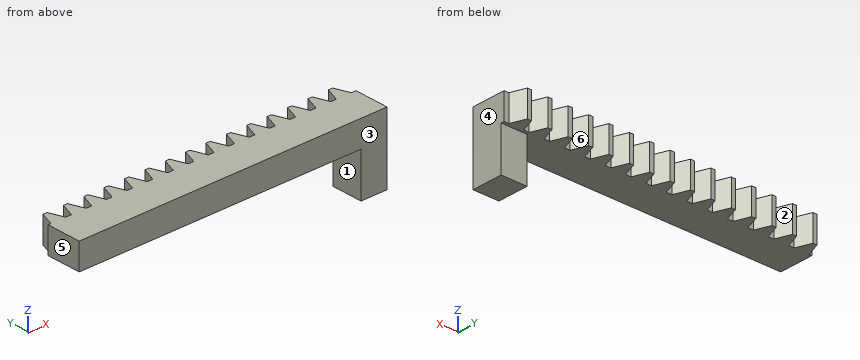
```python
from build123d import *

# Parameters (mm, degrees)
BLANKSKE_W          = 120
BLANKSKE_H          = 16
BLANK_DEPTH         = 8
TOOTHCUTSIM_DEPTH   = 122.326007105
TEETHCUTS_COUNT     = 20
TEETHCUTS_PITCH     = 6.2831853
SKETCH1_W           = 8
SKETCH1_H           = 1
CUT_EXTRUDE1_DEPTH  = 122.326007105
SKETCH2_W           = 13.5
SKETCH2_H           = 9.5
BOSS_EXTRUDE2_DEPTH = 8
CUT_EXTRUDE2_DEPTH  = 123.956293048


with BuildPart() as part:
    # BlankSke → Blank (new body)
    with BuildSketch(Plane.XY):
        with Locations((60, 8)):
            Rectangle(BLANKSKE_W, BLANKSKE_H)
    extrude(amount=-BLANK_DEPTH)

    # TooCutSkeSim → ToothCutSim (cut, through all)
    with BuildSketch(Plane.XY):
        Polygon((0.861870739, 11.5), (-0.861870739, 11.5), (-2.508981637, 16.0254), (2.508981637, 16.0254), align=None)
    toothcutsim = extrude(amount=-TOOTHCUTSIM_DEPTH, mode=Mode.SUBTRACT)

    # TeethCuts: ToothCutSim ×20
    with Locations(*[(i * TEETHCUTS_PITCH, 0, 0) for i in range(1, TEETHCUTS_COUNT)]):
        add(toothcutsim, mode=Mode.SUBTRACT)

    # Sketch1 → Cut-Extrude1 (cut, through all)
    with BuildSketch(Plane(origin=(120, 0, 0), x_dir=(0, 0, -1), z_dir=(1, 0, 0))):
        with Locations((4, 0.5)):
            Rectangle(SKETCH1_W, SKETCH1_H)
    extrude(amount=-CUT_EXTRUDE1_DEPTH, mode=Mode.SUBTRACT)

    # Sketch2 → Boss-Extrude2 (add)
    with BuildSketch(Plane(origin=(120, 0, 0), x_dir=(0, 0, -1), z_dir=(1, 0, 0))):
        with Locations((14.75, 5.75)):
            Rectangle(SKETCH2_W, SKETCH2_H)
    extrude(amount=-BOSS_EXTRUDE2_DEPTH)

    # Sketch3 → Cut-Extrude2 (cut, through all)
    with BuildSketch(Plane.XY):
        with BuildLine():
            Line((0, 1), (0, 11.5))
            ThreePointArc((0, 11.5), (0.43093537, 11.93093537), (0.861870739, 11.5))
            Line((0.861870739, 11.5), (2.499736794, 16))
            Line((2.499736794, 16), (3.783448506, 16))
            Line((3.783448506, 16), (5.421314561, 11.5))
            Line((5.421314561, 11.5), (7.145056039, 11.5))
            Line((7.145056039, 11.5), (8.782922094, 16))
            Line((8.782922094, 16), (10.066633806, 16))
            Line((10.066633806, 16), (11.704499861, 11.5))
            Line((11.704499861, 11.5), (13.428241339, 11.5))
            Line((13.428241339, 11.5), (15.066107394, 16))
            Line((15.066107394, 16), (15.70796325, 16))
            Line((15.70796325, 16), (16.349819106, 16))
            Line((16.349819106, 16), (17.987685161, 11.5))
            Line((17.987685161, 11.5), (19.711426639, 11.5))
            Line((19.711426639, 11.5), (21.349292694, 16))
            Line((21.349292694, 16), (22.633004406, 16))
            Line((22.633004406, 16), (24.270870461, 11.5))
            Line((24.270870461, 11.5), (25.1327412, 11.5))
            Line((25.1327412, 11.5), (25.1327412, 1))
            Line((25.1327412, 1), (17.987685161, 1))
            Line((17.987685161, 1), (15.70796325, 1))
            Line((15.70796325, 1), (6.161314561, 1))
            Line((6.161314561, 1), (0, 1))
        make_face()
    extrude(amount=-CUT_EXTRUDE2_DEPTH, mode=Mode.SUBTRACT)


solid = part.part
```
The listing builds one solid part. Answer for the finished solid, in the listing's coordinates (mm). Face numbers are marked on the shaded views. A direction names the side the tool comes from. Give positions to 0.01 mm unless a question says otherwise; leave off trailing zeros. Order: outer loops, then holes, each group sorted by start corner. A loop starts at its lowest first (then second) coordinate and runs counter-clockwise, first axis right, second up. Notation, with made-up numbers: (15, -6.5) -> (74, -6.5) arc R33 ccw to (74, 24.5) -> close; hole circle Ø8 at (70.25, 8.5). An arc over 180 degrees is marked (long way). Write each question's results on one line, items separated by ' | '.
Q1. The part is cut by section B-B, the plane y = 2.5. Give the vertices of the cut face in (x, z), and give its area (3 significant figures).
Checked values:
outline: (25.13, -8) -> (112, -8) -> (112, -21.5) -> (120, -21.5) -> (120, 0) -> (25.13, 0) -> close | area: 867 mm^2
Q2. Which of the six approach directions +Z, -Z, +X, -X, +Y, -Y give full straight-line access (tool end or side, diameter ignored) to the marked faces 5 and 6?
Checked values:
face 5: +Z, -Z, -X, +Y, -Y | face 6: +Z, -Z, +Y
Q3. Each of these flat-tipped pins is pushed along its axis until it touches: P1, Ø10, axis at x = 35.5, z = -8, coming from the +Y side; P2, Ø4.5, axis at x = 61, y = 8, coming from the -Z side; P3, Ø0.9, axis at x = 113, z = -4.5, coming from the +Y side; P4, Ø2.5, axis at x = 117, z = -14, coming from the +Y side. Where does it stop, or does it pass through?
Checked values:
P1: stops at y = 16 | P2: stops at z = -8 | P3: stops at y = 11.5 | P4: stops at y = 10.5
Q4. The part is cut by section A-A, the plane z = -11. Give the vertices of the cut face in (x, y).
Checked values:
outline: (112, 1) -> (120, 1) -> (120, 10.5) -> (112, 10.5) -> close
Q5. Determine the mould class of the marked faces 1, 2, 3 and 4 for opening direction X: pulls with the +X half, pulls with the -X half, needs draft (parallel to the pull), parting line crosses it, or undercut.
Checked values:
face 1: pulls with the -X half | face 2: undercut | face 3: needs draft | face 4: pulls with the +X half
Q6. Straight lines are drawn through the part: probe 1 along Y at (x, z) = (75, -1); probe 2 along Z at (x, y) = (67, 3.5); probe 3 along X at (y, z) = (6.25, -15.75). For each, find the intervals that lie inside material, in ascending order. Write a range as from..to.
Checked values:
probe 1: y = 1..11.5 | probe 2: z = -8..0 | probe 3: x = 112..120
Q7. The part is cut by section C-C, the plane x = 108.5. Give the vertices of the cut face in (y, z).
Checked values:
outline: (1, -8) -> (13.76, -8) -> (13.76, 0) -> (1, 0) -> close
